Design review of the part built by this model. Coordinates are the model's own, in mm. A direction names the side the tool comes from. Round coordinates to 2 decimals unless told otherwise and drop trailing zeros. Order: outer loops, then holes, each group sorted by start corner. A loop starts at its lowest first (then second) coordinate and runs counter-clockwise, first axis right, second up.
from build123d import *

# Parameters (mm, degrees)
SKETCH_1_W           = 60
SKETCH_1_H           = 5
EXTRUDE_1_DEPTH      = 7
SKETCH_2_W           = 8
SKETCH_2_H           = 5
EXTRUDE_2_DEPTH      = 20
SKETCH_3_R           = 1.5
CUT_EXTRUDE_1_DEPTH  = 15
SKETCH_6_W           = 60
SKETCH_6_H           = 3
EXTRUDE_3_DEPTH      = 35
SKETCH_7_W           = 1
SKETCH_7_H           = 20
CUT_EXTRUDE_2_DEPTH  = 40
SKETCH_8_R           = 1.5
SKETCH_8_R_2         = 7.5
CUT_EXTRUDE_3_DEPTH  = 10
EXTRUDE_4_DEPTH      = 3
EXTRUDE_4_DEPTH_BACK = 9
SKETCH_9_W           = 12
SKETCH_9_H           = 14
SKETCH_9_R           = 2.5
FILLET_3_R           = 3
SKETCH_12_W          = 57.5
SKETCH_12_H          = 5
EXTRUDE_6_DEPTH      = 3
FILLET_6_R           = 3
FILLET_7_R           = 1.5
FILLET_8_R           = 5
FILLET_9_R           = 3
FILLET_10_R          = 3
SKETCH_14_W          = 1.25
SKETCH_14_H          = 5
EXTRUDE_7_DEPTH      = 23
EXTRUDE_8_DEPTH      = 3
FILLET_12_R          = 3
SKETCH_17_R          = 2.6
CUT_EXTRUDE_4_DEPTH  = 15


# Some blends are built 0.0001 mm under size
with BuildPart() as part:
    # 草图1 → 凸台-拉伸1 (new body)
    with BuildSketch(Plane(origin=(0, 0, 0), x_dir=(1, 0, 0), z_dir=(0, 1, 0))):
        Rectangle(SKETCH_1_W, SKETCH_1_H)
    extrude(amount=EXTRUDE_1_DEPTH)

    # 草图2 → 凸台-拉伸2 (add)
    with BuildSketch(Plane(origin=(0, 7, 0), x_dir=(1, 0, 0), z_dir=(0, 1, 0))):
        with Locations((24.75, 0)):
            Rectangle(SKETCH_2_W, SKETCH_2_H)
        with Locations((-24.75, 0)):
            Rectangle(SKETCH_2_W, SKETCH_2_H)
    extrude(amount=EXTRUDE_2_DEPTH)

    # 草图3 → 切除-拉伸1 (cut)
    with BuildSketch(Plane(origin=(0, 0, -2.5), x_dir=(-1, 0, 0), z_dir=(0, 0, -1))):
        with Locations((-24.75, 22)):
            Circle(SKETCH_3_R)
        with Locations((-24.75, 12)):
            Circle(SKETCH_3_R)
        with Locations((24.75, 12)):
            Circle(SKETCH_3_R)
        with Locations((24.75, 22)):
            Circle(SKETCH_3_R)
    extrude(amount=-CUT_EXTRUDE_1_DEPTH, mode=Mode.SUBTRACT)

    # 草图6 → 凸台-拉伸3 (add)
    with BuildSketch(Plane.XY.offset(2.5)):
        with Locations((0, 1.5)):
            Rectangle(SKETCH_6_W, SKETCH_6_H)
    extrude(amount=EXTRUDE_3_DEPTH)

    # 草图7 → 切除-拉伸2 (cut)
    with BuildSketch(Plane(origin=(0, 3, 0), x_dir=(1, 0, 0), z_dir=(0, 1, 0))):
        with Locations((-29.5, -27.5)):
            Rectangle(SKETCH_7_W, SKETCH_7_H)
    extrude(amount=-CUT_EXTRUDE_2_DEPTH, mode=Mode.SUBTRACT)

    # 草图8 → 切除-拉伸3 (cut)
    with BuildSketch(Plane(origin=(0, 3, 0), x_dir=(1, 0, 0), z_dir=(0, 1, 0))):
        with Locations(Location((-25, -19.5, 0), (0, 0, 270))):
            Circle(SKETCH_8_R)
        with Locations(Location((-25, -29.5, 0), (0, 0, 270))):
            Circle(SKETCH_8_R)
        with Locations(Location((26, -29.5, 0), (0, 0, 270))):
            Circle(SKETCH_8_R)
        with Locations(Location((26, -19.5, 0), (0, 0, 270))):
            Circle(SKETCH_8_R)
        with Locations(Location((1, -20.5, 0), (0, 0, 270))):
            Circle(SKETCH_8_R_2)
    extrude(amount=-CUT_EXTRUDE_3_DEPTH, mode=Mode.SUBTRACT)

    # 草图9 → 凸台-拉伸4 (add, two sides: drawn at the far end of the back side and taken through both)
    # profile 1 of 2: a face of its own
    with BuildSketch(Plane(origin=(0, 0, -2.5), x_dir=(-1, 0, 0), z_dir=(0, 0, -1)).offset(-EXTRUDE_4_DEPTH_BACK)):
        with Locations((-16.2, -7)):
            Rectangle(SKETCH_9_W, SKETCH_9_H)
        with Locations((-16.2, -7.219000805)):
            Circle(SKETCH_9_R, mode=Mode.SUBTRACT)
    # profile 2 of 2: a face of its own
    with BuildSketch(Plane(origin=(0, 0, -2.5), x_dir=(-1, 0, 0), z_dir=(0, 0, -1)).offset(-EXTRUDE_4_DEPTH_BACK)):
        with Locations((8.8, -7)):
            Rectangle(SKETCH_9_W, SKETCH_9_H)
        with Locations((8.8, -7.219000805)):
            Circle(SKETCH_9_R, mode=Mode.SUBTRACT)
    extrude(amount=EXTRUDE_4_DEPTH + EXTRUDE_4_DEPTH_BACK)

    # 圆角3
    # the kernel refuses this fillet: 3 mm, written as the material it takes off along each edge
    with BuildSketch(Plane(origin=(-30, 8.590169944, 17.5), x_dir=(0, 0, -1), z_dir=(0, -1, 0))) as fillet_3_piece_1:
        with BuildLine():
            CenterArc((2.236067977, 3), FILLET_3_R, 221.810314896, 48.189685104)
            Line((0, 1), (-0.04472136, 0.96))
            ThreePointArc((-0.04472136, 0.96), (-0.06, 0.5), (-0.06, 0))
            Line((-0.06, 0), (0, -0.06))
            Line((0, -0.06), (2.236067977, -0.06))
            Line((2.236067977, -0.06), (2.236067977, 0))
        make_face()
    extrude(amount=14.180339887, mode=Mode.SUBTRACT)

    # 草图12 → 凸台-拉伸6 (add)
    with BuildSketch(Plane(origin=(0, 27, 0), x_dir=(1, 0, 0), z_dir=(0, 1, 0))):
        Rectangle(SKETCH_12_W, SKETCH_12_H)
    extrude(amount=EXTRUDE_6_DEPTH)

    # 圆角6
    fillet_6_edges = [part.edges().sort_by_distance(p)[0] for p in [
        (-28.75, 30, 0),
        (20.75, 27, 0),
        (-20.75, 27, 0),
    ]]
    fillet(fillet_6_edges, radius=FILLET_6_R)

    # 圆角7
    fillet_7_edges = [part.edges().sort_by_distance(p)[0] for p in [
        (16.2, 0, -2.5),
        (-8.8, 0, -2.5),
    ]]
    fillet(fillet_7_edges, radius=FILLET_7_R)
    fillet_7_2_edges = [part.edges().sort_by_distance(p)[0] for p in [
        (-8.8, 0, -5.5),
        (16.2, 0, -5.5),
    ]]
    fillet(fillet_7_2_edges, radius=FILLET_7_R - 0.0001)  # a hair under: the kernel refuses the full size

    # 圆角8
    fillet_8_edges = [part.edges().sort_by_distance(p)[0] for p in [
        (22.2, 0, 2),
        (10.2, 0, 2),
        (-2.8, 0, 2),
        (-14.8, 0, 2),
    ]]
    fillet(fillet_8_edges, radius=FILLET_8_R)

    # 圆角9
    fillet_9_edges = [part.edges().sort_by_distance(p)[0] for p in [
        (22.2, -14, 0.5),
        (10.2, -14, 0.5),
        (-14.8, -14, 0.5),
        (-2.8, -14, 0.5),
    ]]
    fillet(fillet_9_edges, radius=FILLET_9_R)

    # 圆角10
    fillet_10_edges = [part.edges().sort_by_distance(p)[0] for p in [
        (30, 1.5, 37.5),
        (-29, 1.5, 37.5),
    ]]
    fillet(fillet_10_edges, radius=FILLET_10_R)

    # 草图14 → 凸台-拉伸7 (add)
    with BuildSketch(Plane(origin=(0, 7, 0), x_dir=(1, 0, 0), z_dir=(0, 1, 0))):
        with Locations((29.375, 0)):
            Rectangle(SKETCH_14_W, SKETCH_14_H)
    extrude(amount=EXTRUDE_7_DEPTH)

    # 草图16 → 凸台-拉伸8 (add)
    with BuildSketch(Plane(origin=(30, 0, 0), x_dir=(0, 0, -1), z_dir=(1, 0, 0))):
        Polygon((-12.5, 0), (-12.5, 3), (-2.5, 3), (-2.5, 30), (2.5, 30), (2.5, 0), align=None)
    extrude(amount=EXTRUDE_8_DEPTH)

    # 圆角12
    fillet_12_edges = [part.edges().sort_by_distance(p)[0] for p in [
        (33, 1.5, 12.5),
        (33, 30, 0),
    ]]
    fillet(fillet_12_edges, radius=FILLET_12_R - 0.0001)  # a hair under: the kernel refuses the full size

    # 草图17 → 切除-拉伸4 (cut)
    with BuildSketch(Plane(origin=(0, 0, -5.5), x_dir=(-1, 0, 0), z_dir=(0, 0, -1))):
        with Locations((-16.2, -7.219000805)):
            Circle(SKETCH_17_R)
        with Locations((8.8, -7.219000805)):
            Circle(SKETCH_17_R)
    extrude(amount=-CUT_EXTRUDE_4_DEPTH, mode=Mode.SUBTRACT)


solid = part.part
1) Take a section at A-A on y = 12. Give the boundary of the cut face in (x, z), plus the area to 4 significant figures.
Results:
outline: (-28.75, -2.5) - (-26.25, -2.5) - (-26.25, 2.5) - (-28.75, 2.5) - close; (-23.25, -2.5) - (-20.75, -2.5) - (-20.75, 2.5) - (-23.25, 2.5) - close; (20.75, -2.5) - (23.25, -2.5) - (23.25, 2.5) - (20.75, 2.5) - close; (26.25, -2.5) - (33, -2.5) - (33, 2.5) - (26.25, 2.5) - close
area: 71.25 mm2
2) The part is to be moulded in two halves that separate along Y. For faces 1 (the face through (11.06, -13.1, 0.42)), 2 (the face through (26.25, 12.07, -0.04)), 3 (the face through (-23.25, 12.07, -0.04)), 4 (the face through (-8.88, -0.43, -5.05)), say which applies: released by +Y, released by -Y, zero draft, split by the parting line, or undercut.
Results:
face 1: released by -Y
face 2: undercut
face 3: undercut
face 4: released by +Y
3) Take a section at C-C on z = 30. Give the boundary of the cut face in (x, y), plus the area to 3 significant figures.
Results:
outline: (-29, 0) - (-26.41, 0) - (-26.41, 3) - (-29, 3) - close; (-23.59, 0) - (24.59, 0) - (24.59, 3) - (-23.59, 3) - close; (27.41, 0) - (30, 0) - (30, 3) - (27.41, 3) - close
area: 160 mm2
4) Clearance check with flat-ended pins moving along their axes: P1, Ø1.5, axis at y = -7, z = 5.5, coming from the -X side; P2, Ø2, axis at y = 21, z = 3, coming from the -X side; P3, Ø4, axis at x = -25, z = 19.5, coming from the +Y side; P4, Ø4.5, axis at x = -8.8, y = -7.219, coming from the +Z side. State where each tip first meets the part, or that it passes through.
Results:
P1: stops at x = -14.8
P2: stops at x = -28.75
P3: stops at y = 3
P4: passes through
5) To check wall thickness, follow line 1 along X through (y, z) = (-1.5, -3); line 2 along X through (y, z) = (1.55, 20.5); line 3 along Y through (x, z) = (-9, 4). State the ranges of each line that lie inside material, in increasing order.
Results:
line 1: x = -14.8 to -2.8, 10.2 to 22.2
line 2: x = -29 to -26.12, -23.88 to -6.5, 8.5 to 24.88, 27.12 to 30
line 3: y = -14 to -9.81, -4.63 to 3
6) Take a section at D-D on x = -25. Give the boundary of the cut face in (y, z), plus the area to 3 significant figures.
Results:
outline: (0, -2.5) - (10.52, -2.5) - (10.52, 2.5) - (3, 2.5) - (3, 18) - (0, 18) - close; (0, 21) - (3, 21) - (3, 28) - (0, 28) - close; (0, 31) - (3, 31) - (3, 37.5) - (0, 37.5) - close; (13.48, -2.5) - (20.52, -2.5) - (20.52, 2.5) - (13.48, 2.5) - close; (23.48, -2.5) - (30, -2.5) - (30, 2.5) - (23.48, 2.5) - close
area: 207 mm2
7) Take a section at B-B on x = 16.2. State how many separate pieces and enclosed holes the cut face has, plus the area to 3 significant figures.
Results:
separate pieces: 3
enclosed holes: 0
area: 261 mm2
8) For faces 5 (the face through (-28.75, 17, 0)), 6 (the face through (-14.8, -8, -1)), 7 (the face through (22.2, -8, -1)), 8 (the face through (-29, 2, 26)), 9 (the face through (-3.66, -13.1, 0.42)), list the 3-axis set-ups (+Z, -Z, +X, -X, +Y, -Y) from which the entire face can be reached by the end or side of a thin tool; tool diameter is ignored.
Results:
face 5: +Z, -Z, -X, +Y
face 6: -Z, -X, -Y
face 7: -Z, +X, -Y
face 8: +Z, -X, +Y, -Y
face 9: +Z, -Z, -Y
